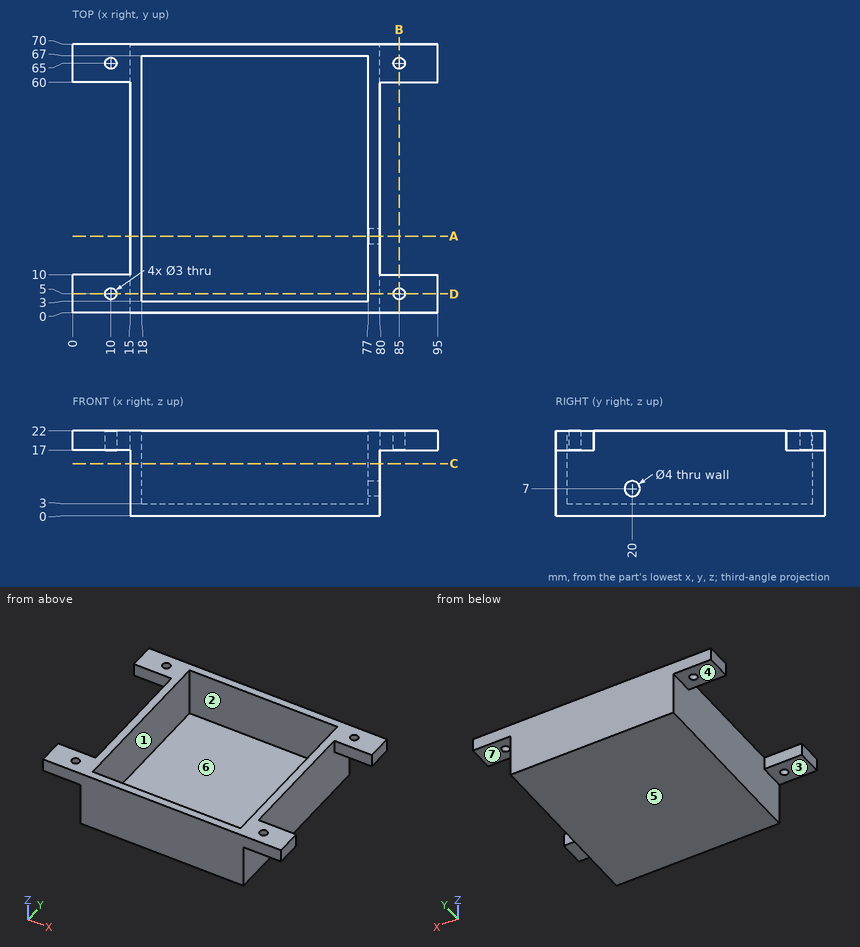
Drawing for the job (mm, zero at the part's lowest x, y, z). A direction names the side the tool comes from. Coordinates: 2 decimals unless noted, no trailing zeros. Order: outer loops, then holes, each group sorted by start corner. A loop starts at its lowest first (then second) coordinate and runs counter-clockwise, first axis right, second up. Notation, with made-up numbers: (42, 84.25) - (67, 84.25) arc R18 cw to (67, 99.25) - close; hole circle Ø5 at (77, -37.5). An arc over 180 degrees is marked (long way). Use a Markdown table: item, result. Add a question column.
(1) Which spindle directions (+Z, -Z, +X, -X, +Y, -Y) get a long thin tool onto all of the face, cutting with end or side? Do the marked faces 4, 5, 6 and 7. Say none if no direction does.
(2) Saw through at D-D (y = 5). Give the cut face in (x, z).
(3) Pull direction X, two halves, no side cores. Call the marked faces 1, 2 and 3: +X half, -X half, draft (parallel to the pull), parting line (faces both ways), or undercut.
(4) Flat gauge pins, fed straight in: pin 1 (2.5 mm diameter, centred on y = 20, z = 7, fed in from +X); pin 2 (5.5 mm diameter, centred on y = 47.5, z = 11.5, fed in from +X); pin 3 (5.5 mm diameter, centred on y = 23, z = 9.5, fed in from -X). Where does each tip first touch, or does it go through?
(5) Drill centre lines: line 1 along Y through (x, z) = (10, 18.6); line 2 along X through (y, z) = (65, 18.3); line 3 along X through (y, z) = (47.5, 20.75). Where is each one in solid material? Low to high. Write a range as [from, to].
(6) Saw through at A-A (y = 20). Give the cut face in (x, z), then the cut area to 3 significant figures.
(7) Saw through at C-C (z = 13.5). Give the cut face in (x, y), then the cut area to 3 significant figures.
(8) Saw through at B-B (x = 85). Give the cut face in (y, z), then the cut area to 3 significant figures.
Solved:
| question | item | result |
|---|---|---|
| 1 | face 4 | -Z, -X, +Y, -Y |
| 1 | face 5 | -Z, +X, -X, +Y, -Y |
| 1 | face 6 | +Z |
| 1 | face 7 | -Z, +X, +Y, -Y |
| 2 | outline | (0, 17) - (8.5, 17) - (8.5, 22) - (0, 22) - close; (11.5, 17) - (15, 17) - (15, 0) - (80, 0) - (80, 17) - (83.5, 17) - (83.5, 22) - (77, 22) - (77, 3) - (18, 3) - (18, 22) - (11.5, 22) - close; (86.5, 17) - (95, 17) - (95, 22) - (86.5, 22) - close |
| 3 | face 1 | undercut |
| 3 | face 2 | undercut |
| 3 | face 3 | draft |
| 4 | pin 1 | stops at x = 18 |
| 4 | pin 2 | stops at x = 80 |
| 4 | pin 3 | stops at x = 15 |
| 5 | line 1 | y = [0, 3.5], [6.5, 10], [60, 63.5], [66.5, 70] |
| 5 | line 2 | x = [0, 8.5], [11.5, 18], [77, 83.5], [86.5, 95] |
| 5 | line 3 | x = [15, 18], [77, 80] |
| 6 | outline | (15, 0) - (80, 0) - (80, 5) - (77, 5) - (77, 3) - (18, 3) - (18, 22) - (15, 22) - close; (77, 9) - (80, 9) - (80, 22) - (77, 22) - close |
| 6 | area | 297 mm² |
| 7 | outline | (15, 0) - (80, 0) - (80, 70) - (15, 70) - close; hole (18, 3) - (77, 3) - (77, 67) - (18, 67) - close |
| 7 | area | 774 mm² |
| 8 | outline | (0, 17) - (3.5, 17) - (3.5, 22) - (0, 22) - close; (6.5, 17) - (10, 17) - (10, 22) - (6.5, 22) - close; (60, 17) - (63.5, 17) - (63.5, 22) - (60, 22) - close; (66.5, 17) - (70, 17) - (70, 22) - (66.5, 22) - close |
| 8 | area | 70.0 mm² |
